```python
from build123d import *

# Parameters (mm, degrees)
CROQUIS1_R              = 21
CROQUIS1_W              = 50
CROQUIS1_H              = 30
SALIENTE_EXTRUIR1_DEPTH = 10
CROQUIS2_R              = 16
CORTAR_EXTRUIR1_DEPTH   = 50.050993874
REDONDEO1_R             = 80
CROQUIS3_R              = 1.5
CORTAR_EXTRUIR2_DEPTH   = 15
MATRIZL1_COUNT          = 2
MATRIZL1_PITCH          = 15
MATRIZL1_COL_COUNT      = 2
MATRIZL1_COL_PITCH      = 15
SKETCH1_R               = 16
BOSS_EXTRUDE1_DEPTH     = 10


with BuildPart() as part:
    # Croquis1 → Saliente-Extruir1 (new body)
    with BuildSketch(Plane(origin=(0, 0, 0), x_dir=(1, 0, 0), z_dir=(0, 1, 0))):
        with Locations((0, 20)):
            Circle(CROQUIS1_R)
        Rectangle(CROQUIS1_W, CROQUIS1_H)
        with BuildLine():
            ThreePointArc((19.296872909, 28.284364546), (0, 41), (-19.296872909, 28.284364546))
            ThreePointArc((-19.296872909, 28.284364546), (-20.928477594, 21.731711756), (-20.396078054, 15))
            Line((-20.396078054, 15), (20.396078054, 15))
            ThreePointArc((20.396078054, 15), (20.848472835, 17.481829944), (21, 20))
            ThreePointArc((21, 20), (20.569811996, 24.228810052), (19.296872909, 28.284364546))
        make_face()
        with BuildLine():
            Line((20.396078054, 15), (-20.396078054, 15))
            ThreePointArc((-20.396078054, 15), (0, -1), (20.396078054, 15))
        make_face()
        with BuildLine():
            Line((25, 15), (19.296872909, 28.284364546))
            ThreePointArc((19.296872909, 28.284364546), (20.569811996, 24.228810052), (21, 20))
            ThreePointArc((21, 20), (20.848472835, 17.481829944), (20.396078054, 15))
            Line((20.396078054, 15), (25, 15))
        make_face()
        with BuildLine():
            Line((-19.296872909, 28.284364546), (-25, 15))
            Line((-25, 15), (-20.396078054, 15))
            ThreePointArc((-20.396078054, 15), (-20.928477594, 21.731711756), (-19.296872909, 28.284364546))
        make_face()
    extrude(amount=SALIENTE_EXTRUIR1_DEPTH)

    # Croquis2 → Cortar-Extruir1 (cut, through all)
    with BuildSketch(Plane(origin=(0, 10, 0), x_dir=(1, 0, 0), z_dir=(0, 1, 0))):
        with Locations(Location((0, 20, 0), (0, 0, 270))):
            Circle(CROQUIS2_R)
    extrude(amount=-CORTAR_EXTRUIR1_DEPTH, mode=Mode.SUBTRACT)

    # Redondeo1
    # the kernel refuses this fillet: 80 mm, written as the material it takes off along each edge
    with BuildSketch(Plane(origin=(25, -40.950006406, -15), x_dir=(-0.39449354980003665, 0, -0.9188987099600074), z_dir=(0, 1, 0))) as redondeo1_piece_1:
        with BuildLine():
            CenterArc((16.50792076, 79.973702153), REDONDEO1_R, 246.765608194, 21.765246915)
            Line((-15.051563224, 6.461805357), (0, 0))
            Line((0, 0), (14.456832295, 0))
        make_face()
    extrude(amount=91.900012811, mode=Mode.SUBTRACT)
    with BuildSketch(Plane(origin=(-25, -40.950006406, -15), x_dir=(0.39449354980003676, 0, -0.9188987099600074), z_dir=(0, 1, 0))) as redondeo1_piece_2:
        with BuildLine():
            CenterArc((16.50792076, -79.973702153), REDONDEO1_R, 91.46914489, 21.765246915)
            Line((-15.051563224, -6.461805357), (0, 0))
            Line((0, 0), (14.456832295, 0))
        make_face()
    extrude(amount=91.900012811, mode=Mode.SUBTRACT)

    # Croquis3 → Cortar-Extruir2 (cut)
    with BuildSketch(Plane.XY.offset(15)):
        with Locations((0, 5)):
            Circle(CROQUIS3_R)
    cortar_extruir2 = extrude(amount=-CORTAR_EXTRUIR2_DEPTH, mode=Mode.SUBTRACT)

    # MatrizL1: Cortar-Extruir2 ×2
    with Locations(*[(i * MATRIZL1_PITCH, 0, 0) for i in range(1, MATRIZL1_COUNT)]):
        add(cortar_extruir2, mode=Mode.SUBTRACT)

    # MatrizL1 col: Cortar-Extruir2 ×2
    with Locations(*[(-i * MATRIZL1_COL_PITCH, 0, 0) for i in range(1, MATRIZL1_COL_COUNT)]):
        add(cortar_extruir2, mode=Mode.SUBTRACT)

    # Sketch1 → Boss-Extrude1 (add)
    with BuildSketch(Plane(origin=(0, 10, 0), x_dir=(1, 0, 0), z_dir=(0, 1, 0))):
        with Locations((0, 20)):
            Circle(SKETCH1_R)
        with BuildLine():
            Line((-2.5, 26.538348415), (-2.5, 29.5))
            Line((-2.5, 29.5), (2.5, 29.5))
            Line((2.5, 29.5), (2.5, 26.538348415))
            ThreePointArc((2.5, 26.538348415), (5.766281297, 23.968626967), (7, 20))
            ThreePointArc((7, 20), (-3.968626967, 14.233718703), (-2.5, 26.538348415))
        make_face(mode=Mode.SUBTRACT)
    extrude(amount=-BOSS_EXTRUDE1_DEPTH)


solid = part.part
```
Read the model definition and answer for the solid it produces. Units are mm, in the model's axes. A direction names the side the tool comes from. Give positions to 0.01 mm unless a question says otherwise; leave off trailing zeros. Write each loop counter-clockwise with the first axis right and the second up, starting at its lowest first coordinate (ties: lowest second). Pieces come first, ordered by that corner, then holes. Notation, with made-up numbers: M 40.25,-17 L 54.25,-17 A22 cw 54.25,17 Z; hole C 56,11.25 d5. An arc over 180 degrees is marked long. Put each result on its own line as item: value. Start each with the question number.
1. Each of these flat-tipped pins is pushed along its axis until it touches: pin 1 Ø3 at (y, z) = (4, -14.5) entering from +X; pin 2 Ø2.5 at (x, y) = (0, 5) entering from +Z; pin 3 Ø2 at (x, y) = (-12.5, 4) entering from -Z. Where does it stop, or does it pass through?
2. Which of the six approach directions +Z, -Z, +X, -X, +Y, -Y give full straight-line access (tool end or side, diameter ignored) to faces 1 (the flat face through (15, 5, 0)), 2 (the cylindrical face through (23.601, 4.93, -13.515)), 3 (the flat face through (-2.5, 5, -28))?
3. Consider line 1 along Y through (x, z) = (15, 4.5); line 2 along X through (y, z) = (4.75, 3); line 3 along X through (y, z) = (3.75, -27). Determine where each line is inside the solid, lowest interval first.
4. The part is cut by section B-B, the plane y = 8.5. Give the vertices of the cut face in (x, z), and give its area (3 significant figures).
5. The part is cut by section C-C, the plane z = -21. Give the vertices of the cut face in (x, y), and give its area (3 significant figures).
6. The part is cut by section A-A, the plane z = 10.5. Give the vertices of the cut face in (x, y).
7. For a pull along X with two mould halves and no side action, classify faces 4 (the flat face through (0, 10, -7)), 5 (the flat face through (0, 5, -29.5)), 6 (the flat face through (25, 5, 8)) as released by +X, released by -X, zero draft, split by the parting line, or undercut.
8. The part is cut by section D-D, the plane y = 5. Give the vertices of the cut face in (x, z).
Final values:
1. pin 1: stops at x = 23.7
1. pin 2: stops at z = 0
1. pin 3: stops at z = -37.57
2. face 1: +Z
2. face 2: -Z, +X, +Y, -Y
2. face 3: +Y, -Y
3. line 1: y = 0 to 3.5, 6.5 to 10
3. line 2: x = -25 to -16.48, -13.52 to -1.48, 1.48 to 13.52, 16.48 to 25
3. line 3: x = -19.8 to -2.5, 2.5 to 19.8
4. outline: M -25,1.38 A80 ccw -19.3,-28.28 A21 ccw 19.3,-28.28 A80 ccw 25,1.38 L 25,15 L -25,15 Z; hole M -2.5,-29.5 L 2.5,-29.5 L 2.5,-26.54 A7 ccw long -2.5,-26.54 Z
4. area: 2,240 mm²
5. outline: M -21.81,0 L -6.93,0 L -6.93,10 L -21.81,10 Z; M 6.93,0 L 21.81,0 L 21.81,10 L 6.93,10 Z
5. area: 298 mm²
6. outline: M -25,0 L 25,0 L 25,10 L -25,10 Z; hole C -15,5 d3; hole C 0,5 d3; hole C 15,5 d3
7. face 4: zero draft
7. face 5: undercut
7. face 6: released by +X
8. outline: M -25,1.38 A80 ccw -19.3,-28.28 A21 ccw 19.3,-28.28 A80 ccw 25,1.38 L 25,15 L 16.5,15 L 16.5,0 L 13.5,0 L 13.5,15 L 1.5,15 L 1.5,0 L -1.5,0 L -1.5,15 L -13.5,15 L -13.5,0 L -16.5,0 L -16.5,15 L -25,15 Z; hole M -2.5,-29.5 L 2.5,-29.5 L 2.5,-26.54 A7 ccw long -2.5,-26.54 Z
